Drawing for the job (mm, zero at the part's lowest x, y, z). Give positions to 0.01 mm unless a question says otherwise; leave off trailing zeros. Order: outer loops, then holes, each group sorted by start corner. A loop starts at its lowest first (then second) coordinate and runs counter-clockwise, first axis right, second up. Notation, with made-up numbers: (30, 82.5) - (67, 82.5) arc R20 cw to (67, 91.5) - close; hole circle Ø7 at (22.5, -30.75). An arc over 180 degrees is marked (long way). One line per item, written item: value.
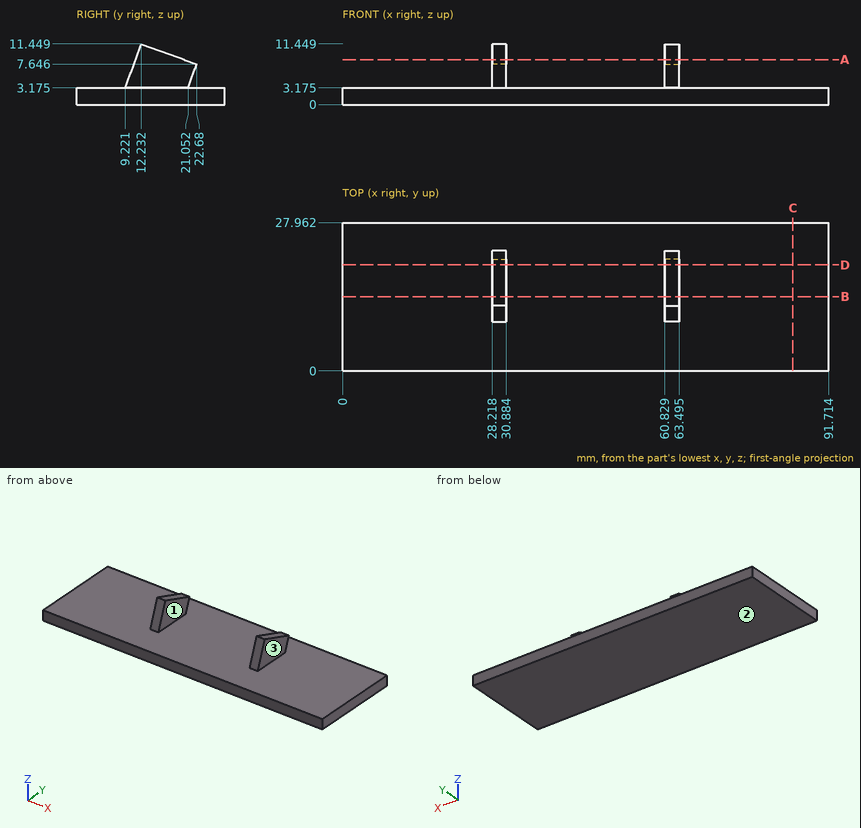
(1) Slice it at B-B, the plane y = 14. Give the cut face in (x, z) (1 decimal).
Completed:
outline: (0, 0) - (91.7, 0) - (91.7, 3.2) - (63.5, 3.2) - (63.5, 10.8) - (60.8, 10.8) - (60.8, 3.2) - (30.9, 3.2) - (30.9, 10.8) - (28.2, 10.8) - (28.2, 3.2) - (0, 3.2) - close
(2) Pin check, flat tips, straight feed: P1, Ø12, axis at x = 51, y = 9, coming from the +Z side (1 decimal); P2, Ø6.5, axis at y = 14.5, z = 6.5, coming from the +X side (1 decimal); P3, Ø4, axis at y = 19, z = 6.5, coming from the -X side. Stop position of each tip, or through.
Completed:
P1: z = 3.2
P2: x = 63.5
P3: x = 28.22
(3) Slice it at C-C, the plane x = 85. Give the cut face in (y, z) (1 decimal).
Completed:
outline: (0, 0) - (28, 0) - (28, 3.2) - (0, 3.2) - close
(4) Drill centre lines: line 1 (X direction, y = 18.25, z = 7) (1 decimal); line 2 (Z direction, x = 49, y = 21.5) (1 decimal); line 3 (Z direction, x = 61.5, y = 21). Where is each one in solid material? Low to high.
Completed:
line 1: 28.2 to 30.9, 60.8 to 63.5
line 2: 0 to 3.2
line 3: 0 to 8.26
(5) Pull direction X, two halves, no side cores. Call the marked faces 1, 2 and 3: +X half, -X half, draft (parallel to the pull), parting line (faces both ways), or undercut.
Completed:
face 1: undercut
face 2: draft
face 3: +X half
(6) Slice it at A-A, the plane z = 8.5. Give the cut face in (x, y) (1 decimal).
Completed:
outline: (28.2, 11.2) - (30.9, 11.2) - (30.9, 20.3) - (28.2, 20.3) - close; (60.8, 11.2) - (63.5, 11.2) - (63.5, 20.3) - (60.8, 20.3) - close
(7) Slice it at D-D, the plane y = 20. Give the cut face in (x, z) (1 decimal).
Completed:
outline: (0, 0) - (91.7, 0) - (91.7, 3.2) - (63.5, 3.2) - (63.5, 8.6) - (60.8, 8.6) - (60.8, 3.2) - (30.9, 3.2) - (30.9, 8.6) - (28.2, 8.6) - (28.2, 3.2) - (0, 3.2) - close
